Read the model definition and answer for the solid it produces. Units are mm, in the model's axes. Face numbers are marked on the shaded views. A direction names the side the tool comes from. Coordinates: 2 decimals unless noted, no trailing zeros. Write each loop counter-clockwise with the first axis right and the second up, starting at its lowest first coordinate (ties: lowest second). Pieces come first, ordered by that corner, then holes. Notation, with made-up numbers: (15.25, 21) -> (66.25, 21) arc R26 cw to (66.25, 47) -> close; hole circle Ø5 at (69.25, -6.5). An arc over 180 degrees is marked (long way). Answer in a Markdown table with one row per item. Add a question column.
Item 1: For a pull along Z with two mould halves and no side action, classify the marked faces 1, 2, 3 and 4 as +Z half, -Z half, draft (parallel to the pull), parting line (faces both ways), or undercut.
Item 2: Which of the six approach directions +Z, -Z, +X, -X, +Y, -Y give full straight-line access (tool end or side, diameter ignored) to the marked faces 5, 6 and 7?
Item 3: Given pin 1 Ø11 at (x, z) = (-40, 0) entering from +Y; pin 2 Ø7.5 at (y, z) = (45, 1.5) entering from -X; pin 3 Ø3 at (x, z) = (-23, 14.5) entering from +Y, each flat-ended and moving along its own axis, determine where each tip first touches the part or whether it passes through.
Item 4: Section C-C on z = -16.5 is taken. Write down the section's boundary in (x, y).
Item 5: Straight lines are drawn through the part: line 1 (Z direction, x = -3.5, y = 40); line 2 (X direction, y = 6, z = 0); line 3 (X direction, y = 35.5, z = 2.5). For each, find the intervals that lie inside material, in ascending order. Write a range as from..to.
Item 6: Section A-A on z = 0 is taken. Write down the section's boundary in (x, y).
Item 7: Section B-B on y = 23.5 is taken. Write down the section's boundary in (x, z), then the cut area to 3 significant figures.
Item 8: Section D-D on x = -22.5 is taken. Write down the section's boundary in (y, z), then the cut area to 3 significant figures.
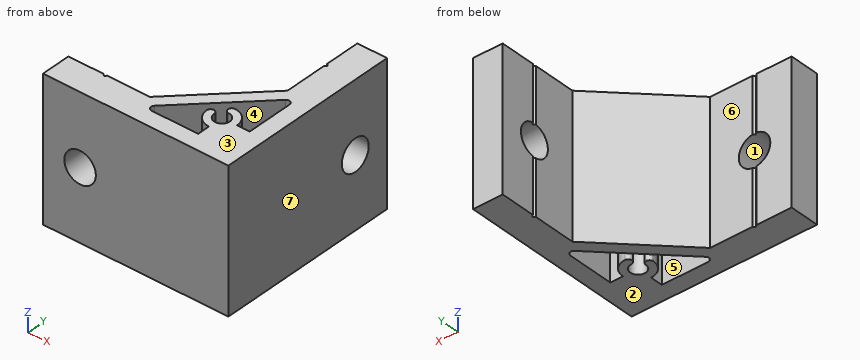
```python
from build123d import *

# Parameters (mm, degrees)
EXTRUDE_1_DEPTH     = 19
SKETCH_2_R          = 4.25
CUT_EXTRUDE_1_DEPTH = 9
SKETCH_3_R          = 4.25
CUT_EXTRUDE_2_DEPTH = 9


with BuildPart() as part:
    # Эскиз1 → Бобышка-Вытянуть1 (new body, symmetric)
    with BuildSketch(Plane.XY):
        Polygon((-50, 0), (0, 0), (0, 50), (-8, 50), (-8, 40.5), (-7.5, 40), (-8, 39.5), (-8, 28), (-28, 8), (-39.5, 8), (-40, 7.5), (-40.5, 8), (-50, 8), align=None)
        with BuildLine():
            Line((-4.5, 12), (-4.5, 24.560303038))
            ThreePointArc((-4.5, 24.560303038), (-5.117316568, 25.484182571), (-6.207106781, 25.267409819))
            Line((-6.207106781, 25.267409819), (-25.267409819, 6.207106781))
            ThreePointArc((-25.267409819, 6.207106781), (-25.484182571, 5.117316568), (-24.560303038, 4.5))
            Line((-24.560303038, 4.5), (-12, 4.5))
            Line((-12, 4.5), (-12, 7.9))
            ThreePointArc((-12, 7.9), (-14.899137803, 9.100862197), (-16.1, 12))
            ThreePointArc((-16.1, 12), (-15.1, 13), (-14.1, 12))
            ThreePointArc((-14.1, 12), (-10.51507576, 10.51507576), (-12, 14.1))
            ThreePointArc((-12, 14.1), (-13, 15.1), (-12, 16.1))
            ThreePointArc((-12, 16.1), (-9.100862197, 14.899137803), (-7.9, 12))
            Line((-7.9, 12), (-4.5, 12))
        make_face(mode=Mode.SUBTRACT)
    extrude(amount=EXTRUDE_1_DEPTH, both=True)

    # Эскиз2 → Вырез-Вытянуть1 (cut, through all)
    with BuildSketch(Plane.ZY.offset(8)):
        with Locations(Location((0, 40, 0), (0, 0, 270))):  # turned: the seam where the file's is
            Circle(SKETCH_2_R)
    extrude(amount=-CUT_EXTRUDE_1_DEPTH, mode=Mode.SUBTRACT)

    # Эскиз3 → Вырез-Вытянуть2 (cut, through all)
    with BuildSketch(Plane(origin=(0, 8, 0), x_dir=(1, 0, 0), z_dir=(0, 1, 0))):
        with Locations(Location((-40, 0, 0), (0, 0, 180))):  # turned: the seam where the file's is
            Circle(SKETCH_3_R)
    extrude(amount=-CUT_EXTRUDE_2_DEPTH, mode=Mode.SUBTRACT)


solid = part.part
```
Results below:
| question | item | result |
|---|---|---|
| 1 | face 1 | undercut |
| 1 | face 2 | -Z half |
| 1 | face 3 | +Z half |
| 1 | face 4 | draft |
| 2 | face 5 | +Z, -Z |
| 2 | face 6 | +Z, -Z, -X, +Y |
| 2 | face 7 | +Z, -Z, +X, +Y, -Y |
| 3 | pin 1 | stops at y = 8 |
| 3 | pin 2 | stops at x = -8 |
| 3 | pin 3 | stops at y = 14.5 |
| 4 | outline | (-50, 0) -> (0, 0) -> (0, 50) -> (-8, 50) -> (-8, 40.5) -> (-7.5, 40) -> (-8, 39.5) -> (-8, 28) -> (-28, 8) -> (-39.5, 8) -> (-40, 7.5) -> (-40.5, 8) -> (-50, 8) -> close; hole (-25.27, 6.21) arc R1 ccw to (-24.56, 4.5) -> (-12, 4.5) -> (-12, 7.9) arc R4.1 cw to (-16.1, 12) arc R1 cw to (-14.1, 12) arc R2.1 ccw (long way) to (-12, 14.1) arc R1 cw to (-12, 16.1) arc R4.1 cw to (-7.9, 12) -> (-4.5, 12) -> (-4.5, 24.56) arc R1 ccw to (-6.21, 25.27) -> close |
| 5 | line 1 | z = -19..-4.25, 4.25..19 |
| 5 | line 2 | x = -50..-44.25, -35.75..-25.43, -12..0 |
| 5 | line 3 | x = -8..0 |
| 6 | outline | (-50, 0) -> (-44.25, 0) -> (-44.25, 8) -> (-50, 8) -> close; (-35.75, 0) -> (0, 0) -> (0, 35.75) -> (-8, 35.75) -> (-8, 28) -> (-28, 8) -> (-35.75, 8) -> close; (-8, 44.25) -> (0, 44.25) -> (0, 50) -> (-8, 50) -> close; hole (-25.27, 6.21) arc R1 ccw to (-24.56, 4.5) -> (-12, 4.5) -> (-12, 7.9) arc R4.1 cw to (-16.1, 12) arc R1 cw to (-14.1, 12) arc R2.1 ccw (long way) to (-12, 14.1) arc R1 cw to (-12, 16.1) arc R4.1 cw to (-7.9, 12) -> (-4.5, 12) -> (-4.5, 24.56) arc R1 ccw to (-6.21, 25.27) -> close |
| 7 | outline | (-12.5, -19) -> (-7.97, -19) -> (-7.97, 19) -> (-12.5, 19) -> close; (-4.5, -19) -> (0, -19) -> (0, 19) -> (-4.5, 19) -> close |
| 7 | area | 343 mm2 |
| 8 | outline | (0, -19) -> (4.5, -19) -> (4.5, 19) -> (0, 19) -> close; (8.97, -19) -> (13.5, -19) -> (13.5, 19) -> (8.97, 19) -> close |
| 8 | area | 343 mm2 |
